The model under review builds one solid part; all positions refer to its coordinate system, in mm. A direction names the side the tool comes from. Coordinates: 2 decimals unless noted, no trailing zeros. Write each loop counter-clockwise with the first axis right and the second up, starting at its lowest first coordinate (ties: lowest second). Pieces come first, ordered by that corner, then holes. Notation, with made-up numbers: (83.25, -10) - (108.25, -10) arc R22 ccw to (108.25, 22) - close; hole circle Ø11 at (2.25, -24). An arc over 180 degrees is marked (long way). Return JSON: item names as keys, results as strings. Group by question number.
(1) Draft analysis for pull direction Z (two halves, no side actions). For faces 3 (the face through (1, 6, -50)), 4 (the face through (1, 6, 50)), 5 (the face through (66.703, 6.058, 48.435)), 6 (the face through (-97.3, 0, -24.9)), state which applies: released by +Z, released by -Z, zero draft, split by the parting line, or undercut.
(2) We need section C-C on x = -42.5. State the section outline as (y, z) points (1 decimal), then the cut area to 3 significant figures.
(3) For pin 1 Ø7.5 at (x, z) = (-94, -25) entering from +Y; pin 2 Ø10.5 at (x, z) = (94, -25) entering from -Y, all flat-tipped, find the tip position at first contact; note any pin that passes through.
(4) Tool access review of faces 1 (the face through (100, 1, 0)), 2 (the face through (1, 8, -46.825)): name each direction out of +Z, -Z, +X, -X, +Y, -Y from which nothing blocks a thin tool from reaching the whole face with its end or side.
(5) We need section D-D on z = 40. State the section outline as (x, y) points, then the cut area to 3 significant figures.
(6) We need section A-A on z = 1. State the section outline as (x, y) points, then the cut area to 3 significant figures.
(7) To check wall thickness, follow L1, parallel to Z at x = -94, y = -0.3; L2, parallel to Z at x = -36, y = 6.75 (3 decimals); L3, parallel to Y at x = -70, z = 49. State the ranges of each line that lie inside material, in increasing order. Write a range as from..to.
(8) We need section B-B on x = 94. State the section outline as (y, z) points (1 decimal).
```python
from build123d import *

# Parameters (mm, degrees)
F1_DEPTH      = 100
F2_W          = 16
F2_H          = 8
F2_R          = 3.3
F3_DEPTH      = 228
F3_DEPTH_BACK = 15.001
F4_R          = 3.3
F5_DEPTH      = 100.001
F6_R          = 7.9375
F7_DEPTH      = 15.001


# Not quite as in the source:
# - an extrude ends at something that could not be found from the text; its depth is read off the source's solid


with BuildPart() as f1:
    # F0 (on Right) → F1 (new body, symmetric)
    with BuildSketch(Plane.YZ):
        Polygon((13.4125, 50), (1.5875, 50), (-1.5875, 50), (-1.5875, 46.825), (-1.5875, -46.825), (-1.5875, -50), (1.5875, -50), (13.4125, -50), (13.4125, -46.825), (1.5875, -46.825), (1.5875, 46.825), (13.4125, 46.825), align=None)
    extrude(amount=F1_DEPTH, both=True)

    # F2 (on face) → F3 (cut, two sides)
    with BuildSketch(Plane.XZ.offset(1.5875)) as f3_sk:
        Rectangle(F2_W, F2_H)
        with Locations((94, -25)):
            Circle(F2_R)
        with Locations((94, 25)):
            Circle(F2_R)
        with Locations((-94, -25)):
            Circle(F2_R)
        with Locations((-94, 25)):
            Circle(F2_R)
    extrude(amount=F3_DEPTH, mode=Mode.SUBTRACT)
    extrude(f3_sk.sketch, amount=-F3_DEPTH_BACK, mode=Mode.SUBTRACT)

    # F4 (on face) → F5 (cut, through all)
    with BuildSketch(Plane.XY.offset(50)):
        with Locations((-70, 5.9125)):
            Circle(F4_R)
        with Locations((70, 5.9125)):
            Circle(F4_R)
    extrude(amount=-F5_DEPTH, mode=Mode.SUBTRACT)

    # F6 (on face) → F7 (cut, through all)
    with BuildSketch(Plane.XZ.offset(1.5875)):
        with Locations((47.8418069781, 24.1387402225)):
            Circle(F6_R)
    extrude(amount=-F7_DEPTH, mode=Mode.SUBTRACT)


solid = f1.part
```
Ans:
{
 "1": {"face 3": "released by -Z", "face 4": "released by +Z", "face 5": "zero draft", "face 6": "undercut"},
 "2": {"outline": "(-1.6, -50) - (13.4, -50) - (13.4, -46.8) - (1.6, -46.8) - (1.6, 46.8) - (13.4, 46.8) - (13.4, 50) - (-1.6, 50) - close", "area": "393 mm²"},
 "3": {"pin 1": "y = 1.59", "pin 2": "y = -1.59"},
 "4": {"face 1": "+Z, -Z, +X, +Y, -Y", "face 2": "+X, -X, +Y"},
 "5": {"outline": "(-100, -1.59) - (100, -1.59) - (100, 1.59) - (-100, 1.59) - close", "area": "635 mm²"},
 "6": {"outline": "(-100, -1.59) - (-8, -1.59) - (-8, 1.59) - (-100, 1.59) - close; (8, -1.59) - (100, -1.59) - (100, 1.59) - (8, 1.59) - close", "area": "584 mm²"},
 "7": {"L1": "-50..-28.3, -21.7..21.7, 28.3..50", "L2": "-50..-46.825, 46.825..50", "L3": "-1.59..2.61, 9.21..13.41"},
 "8": {"outline": "(-1.6, -50) - (13.4, -50) - (13.4, -46.8) - (1.6, -46.8) - (1.6, -28.3) - (-1.6, -28.3) - close; (-1.6, -21.7) - (1.6, -21.7) - (1.6, 21.7) - (-1.6, 21.7) - close; (-1.6, 28.3) - (1.6, 28.3) - (1.6, 46.8) - (13.4, 46.8) - (13.4, 50) - (-1.6, 50) - close"}
}
